The model under review builds one solid part; all positions refer to its coordinate system, in mm. Face numbers are marked on the shaded views. Round coordinates to 2 decimals unless told otherwise and drop trailing zeros. Write each loop counter-clockwise with the first axis right and the second up, starting at its lowest first coordinate (ties: lowest second). Pieces come first, ordered by that corner, then holes.
Item 1: Add section A-A (x = 9.75). Give the boundary of the cut face in (y, z), plus the area to 3 significant figures.
Item 2: Clearance check with flat-ended pins moving along their axes: pin 1 Ø6 at (x, y) = (7, 8.5) entering from +Z; pin 2 Ø1.6 at (x, y) = (1, 9) entering from +Z; pin 3 Ø0.6 at (x, z) = (7.5, 1) entering from +Y. State where each tip first meets the part, or that it passes through.
Item 3: Draft analysis for pull direction Z (two halves, no side actions). For the marked faces 1 and 2, state which applies: +Z half, -Z half, draft (parallel to the pull), parting line (faces both ways), or undercut.
Item 4: To check wall thickness, follow L1, parallel to X at y = 1.15, z = 82.5; L2, parallel to X at y = 3.5, z = 24.5. State the ranges of each line that lie inside material, in increasing order.
Item 5: Add section C-C (z = 82.5). Give the boundary of the cut face in (x, y), plus the area to 3 significant figures.
Item 6: Add section D-D (z = 61.5). Give the boundary of the cut face in (x, y).
Item 7: Add section B-B (y = 11). Give the boundary of the cut face in (x, z).
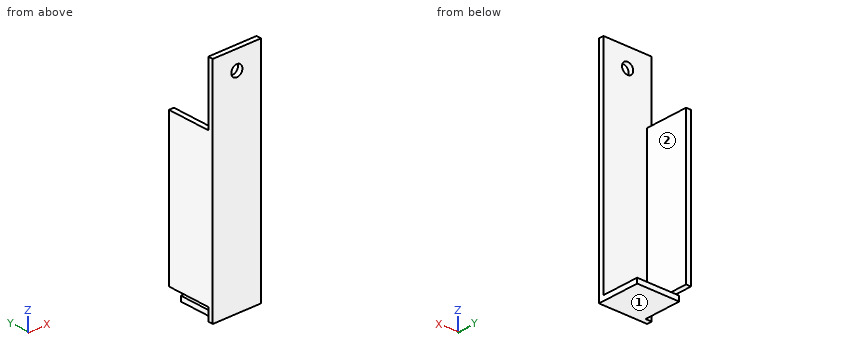
```python
from build123d import *

# Parameters (mm, degrees)
BOSS_EXTRUDE1_DEPTH = 90
SKETCH8_W           = 25
SKETCH8_H           = 17.5
SKETCH8_W_2         = 5
CUT_EXTRUDE1_DEPTH  = 94.736332337
SKETCH2_W           = 17
SKETCH2_H           = 2
BOSS_EXTRUDE2_DEPTH = 15
SKETCH9_R           = 2.25
CUT_EXTRUDE2_DEPTH  = 94.736332337


with BuildPart() as part:
    # Sketch1 → Boss-Extrude1 (new body)
    with BuildSketch(Plane.XY):
        Polygon((0, 0), (0, 19.5), (2, 19.5), (2, 2), (19.5, 2), (19.5, 0), align=None)
    extrude(amount=BOSS_EXTRUDE1_DEPTH)

    # Sketch8 → Cut-Extrude1 (cut, through all)
    with BuildSketch(Plane(origin=(2, 0, 0), x_dir=(0, 0, -1), z_dir=(1, 0, 0))):
        with Locations((-77.5, 10.75)):
            Rectangle(SKETCH8_W, SKETCH8_H)
        with Locations((-2.5, 10.75)):
            Rectangle(SKETCH8_W_2, SKETCH8_H)
    extrude(amount=-CUT_EXTRUDE1_DEPTH, mode=Mode.SUBTRACT)

    # Sketch2 → Boss-Extrude2 (add)
    with BuildSketch(Plane(origin=(0, 2, 0), x_dir=(1, 0, 0), z_dir=(0, 1, 0))):
        with Locations((11, -1)):
            Rectangle(SKETCH2_W, SKETCH2_H)
    extrude(amount=BOSS_EXTRUDE2_DEPTH)

    # Sketch9 → Cut-Extrude2 (cut, through all)
    with BuildSketch(Plane(origin=(0, 2, 0), x_dir=(1, 0, 0), z_dir=(0, 1, 0))):
        with Locations(Location((9.75, -82.5, 0), (0, 0, 270))):
            Circle(SKETCH9_R)
    extrude(amount=-CUT_EXTRUDE2_DEPTH, mode=Mode.SUBTRACT)


solid = part.part
```
Numbers:
1. outline: (0, 0) - (17, 0) - (17, 2) - (2, 2) - (2, 80.25) - (0, 80.25) - close; (0, 84.75) - (2, 84.75) - (2, 90) - (0, 90) - close
1. area: 201 mm2
2. pin 1: stops at z = 2
2. pin 2: stops at z = 65
2. pin 3: stops at y = 17
3. face 1: -Z half
3. face 2: draft
4. L1: x = 0 to 7.5, 12 to 19.5
4. L2: x = 0 to 2
5. outline: (0, 0) - (7.5, 0) - (7.5, 2) - (0, 2) - close; (12, 0) - (19.5, 0) - (19.5, 2) - (12, 2) - close
5. area: 30.0 mm2
6. outline: (0, 0) - (19.5, 0) - (19.5, 2) - (2, 2) - (2, 19.5) - (0, 19.5) - close
7. outline: (0, 5) - (2, 5) - (2, 65) - (0, 65) - close; (2.5, 0) - (19.5, 0) - (19.5, 2) - (2.5, 2) - close
